The drawing under review shows one solid part. Ordinate dimensions are in mm from its lowest x, y, z. Coordinates: 2 decimals unless noted, no trailing zeros. Order: outer loops, then holes, each group sorted by start corner. A loop starts at its lowest first (then second) coordinate and runs counter-clockwise, first axis right, second up.
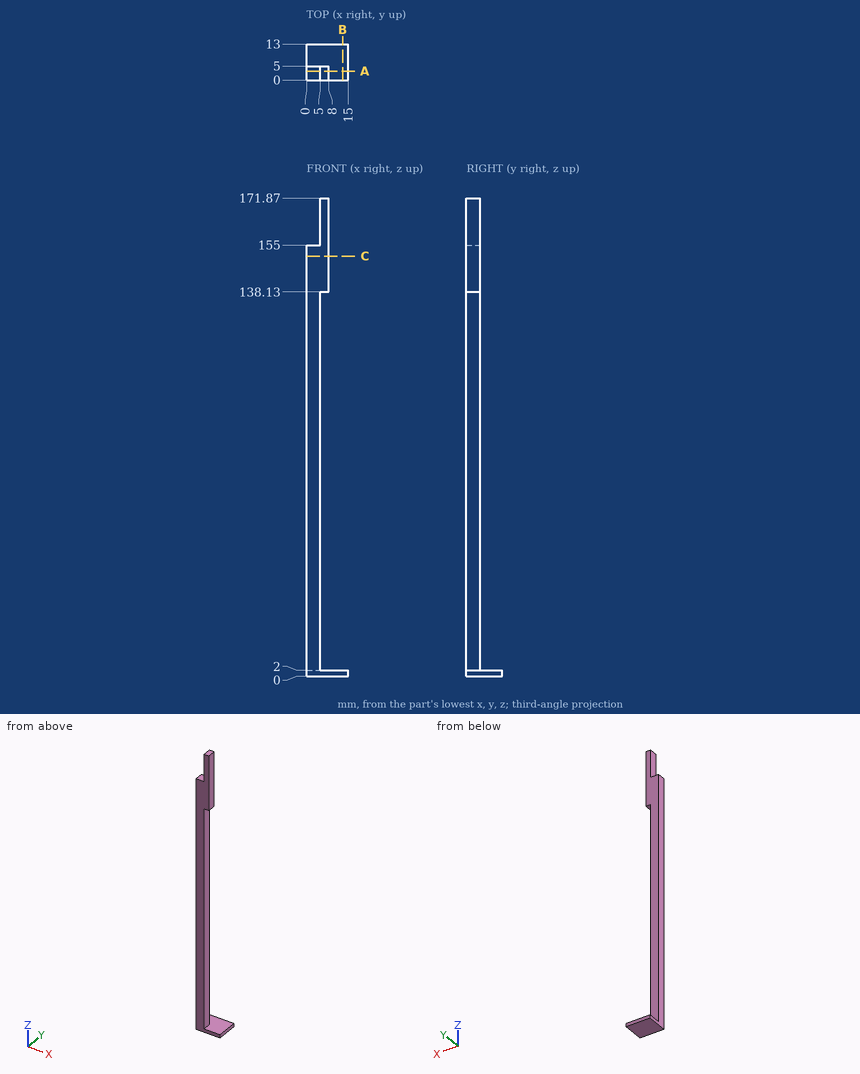
1. To check wall thickness, follow L1, parallel to Z at x = 7.5, y = 3; L2, parallel to X at y = 1.5, z = 65; L3, parallel to Z at x = 3.25, y = 6.25. State the ranges of each line that lie inside material, in increasing order.
Answer below:
L1: z = 0 to 2, 138.13 to 171.87
L2: x = 0 to 5
L3: z = 0 to 2
2. Take a section at C-C, the plane z = 151. Give the boundary of the cut face in (x, y), plus the area to 3 significant figures.
Answer below:
outline: (0, 0) - (8, 0) - (8, 5) - (0, 5) - close
area: 40.0 mm2
3. Take a section at A-A, the plane y = 3.25. Give the boundary of the cut face in (x, z).
Answer below:
outline: (0, 0) - (15, 0) - (15, 2) - (5, 2) - (5, 138.13) - (8, 138.13) - (8, 171.87) - (5, 171.87) - (5, 155) - (0, 155) - close
4. Clearance check with flat-ended pins moving along their axes: pin 1 Ø5.5 at (y, z) = (2.5, 162.5) entering from -X; pin 2 Ø2.5 at (x, z) = (5.5, 106) entering from +Y; pin 3 Ø5.5 at (y, z) = (3.5, 151.5) entering from +X. State where each tip first meets the part, or that it passes through.
Answer below:
pin 1: stops at x = 5
pin 2: stops at y = 5
pin 3: stops at x = 8
5. Take a section at B-B, the plane x = 13. Give the boundary of the cut face in (y, z).
Answer below:
outline: (0, 0) - (13, 0) - (13, 2) - (0, 2) - close
